Work out the finished part from the listing and answer in its coordinate system (mm). Coordinates: 2 decimals unless noted, no trailing zeros. Write each loop counter-clockwise with the first axis right and the second up, starting at its lowest first coordinate (ties: lowest second). Pieces come first, ordered by that corner, then holes. Notation, with made-up numbers: (8.25, 61) - (58.25, 61) arc R18 ccw to (58.25, 66) - close; hole circle Ø6 at (38.25, 46.5). An arc over 180 degrees is marked (long way). One line per item, written item: value.
```python
from build123d import *

# Parameters (mm, degrees)
SKETCH1_W           = 310
SKETCH1_H           = 100
BOSS_EXTRUDE1_DEPTH = 4
SCALE1_SCALE        = 0.5


with BuildPart() as part:
    # Sketch1 → Boss-Extrude1 (new body)
    with BuildSketch(Plane(origin=(0, 0, 0), x_dir=(1, 0, 0), z_dir=(0, 1, 0))):
        Polygon((155, -100), (0, -100), (155, -160), align=None)
        with Locations((155, -50)):
            Rectangle(SKETCH1_W, SKETCH1_H)
        Polygon((155, -100), (155, -160), (310, -100), align=None)
    extrude(amount=BOSS_EXTRUDE1_DEPTH)


with BuildPart() as part_1:
    # Scale1: scaled about (155, 2, 66.153846154)
    add(part.part.scale(SCALE1_SCALE).moved(Location((77.5, 1, 33.076923077))))


solid = part_1.part
```
Item 1: Section A-A, the plane y = 1.75 is taken. Determine the outline of the cut face in (x, z).
Evaluation:
outline: (77.5, 33.08) - (232.5, 33.08) - (232.5, 83.08) - (155, 113.08) - (77.5, 83.08) - close
Item 2: Consider probe 1 along Z at (x, y) = (146.5, 2.7); probe 2 along Z at (x, y) = (199, 1.85). Determine where each line is inside the solid, lowest interval first.
Evaluation:
probe 1: z = 33.08 to 109.79
probe 2: z = 33.08 to 96.04
Item 3: Section C-C, the plane z = 105.5 is taken. Determine the outline of the cut face in (x, y).
Evaluation:
outline: (135.43, 1) - (174.57, 1) - (174.57, 3) - (135.43, 3) - close
Item 4: Section B-B, the plane x = 151.5 is taken. Determine the outline of the cut face in (y, z), then the cut area to 3 significant figures.
Evaluation:
outline: (1, 33.08) - (3, 33.08) - (3, 111.72) - (1, 111.72) - close
area: 157 mm2
